CAD build for the part. Positions are in the model's coordinates, mm. A direction names the side the tool comes from. Coordinates: 2 decimals unless noted, no trailing zeros. Order: outer loops, then holes, each group sorted by start corner. A loop starts at its lowest first (then second) coordinate and runs counter-clockwise, first axis right, second up. Notation, with made-up numbers: M 23,9 L 61,9 A20 cw 61,27 Z; hole C -20,71.5 d5. An arc over 180 degrees is marked long. One line per item, written item: value.
from build123d import *

# Parameters (mm, degrees)
F3_D      = 3.3
F3_DEPTH  = 7
F3_TIP    = 0.9914200214
F4_R      = 10
F4_R_2    = 5
F5_DEPTH  = 9.5
F6_SIZE   = 2.5
F8_DEPTH  = 17
F10_D     = 3.3
F10_DEPTH = 5.2
F10_TIP   = 0.9914200214
F11_R     = 4
F12_DEPTH = 0.5
F14_D     = 3.3
F14_DEPTH = 5.2
F14_TIP   = 0.9914200214
F15_R     = 4
F16_DEPTH = 0.5


with BuildPart() as f1:
    # F0 (on Front) → F1 (revolve)
    with BuildSketch(Plane.XZ):
        Polygon((-20, 4), (0, 4), (0, 13), (-18, 13), (-18, 6), (-20, 6), align=None)
    revolve(axis=Axis((-7.6375159387, 0, 0), (-1, 0, 0)))

    # F3
    with Locations(Plane(origin=(-18, 0, 0), x_dir=(0, -1, 0), z_dir=(-1, 0, 0))):
        with Locations((-7, 7), (7, 7), (-7, -7), (7, -7)):
            Hole(F3_D / 2, depth=F3_DEPTH)
            with Locations((0, 0, -(F3_DEPTH + F3_TIP / 2))):  # 118° drill point
                Cone(0, F3_D / 2, F3_TIP, mode=Mode.SUBTRACT)

    # F4 (on face) → F5 (join)
    with BuildSketch(Plane.YZ):
        Circle(F4_R)
        Circle(F4_R_2, mode=Mode.SUBTRACT)
    extrude(amount=F5_DEPTH)

    # F6
    f6_edges = [f1.edges().sort_by_distance(p)[0] for p in [
        (9.5, -10, 0),
    ]]
    chamfer(f6_edges, length=F6_SIZE)

    # F7 (on face) → F8 (cut)
    with BuildSketch(Plane(origin=(-18, 0, 0), x_dir=(0, -1, 0), z_dir=(-1, 0, 0))):
        with BuildLine():
            Line((-4, 12.3693168769), (4, 12.3693168769))
            ThreePointArc((4, 12.3693168769), (0, 13), (-4, 12.3693168769))
        make_face()
        with BuildLine():
            Line((4, -12.3693168769), (-4, -12.3693168769))
            ThreePointArc((-4, -12.3693168769), (0, -13), (4, -12.3693168769))
        make_face()
    extrude(amount=-F8_DEPTH, mode=Mode.SUBTRACT)

    # F10
    with Locations(Plane.XY.offset(12.3693168769)):
        with Locations((-7, 0)):
            Hole(F10_D / 2, depth=F10_DEPTH)
            with Locations((0, 0, -(F10_DEPTH + F10_TIP / 2))):  # 118° drill point
                Cone(0, F10_D / 2, F10_TIP, mode=Mode.SUBTRACT)

    # F11 (on face) → F12 (cut)
    with BuildSketch(Plane.XY.offset(12.3693168769)):
        with Locations((-7, 0)):
            Circle(F11_R)
    extrude(amount=-F12_DEPTH, mode=Mode.SUBTRACT)

    # F14
    with Locations(Plane(origin=(0, 0, -12.3693168769), x_dir=(1, 0, 0), z_dir=(0, 0, -1))):
        with Locations((-7, -0.0519943278)):
            Hole(F14_D / 2, depth=F14_DEPTH)
            with Locations((0, 0, -(F14_DEPTH + F14_TIP / 2))):  # 118° drill point
                Cone(0, F14_D / 2, F14_TIP, mode=Mode.SUBTRACT)

    # F15 (on face) → F16 (cut)
    with BuildSketch(Plane(origin=(0, 0, -12.3693168769), x_dir=(1, 0, 0), z_dir=(0, 0, -1))):
        with Locations((-7, -0.0519943278)):
            Circle(F15_R)
    extrude(amount=-F16_DEPTH, mode=Mode.SUBTRACT)


solid = f1.part
Q1. Drill centre lines: line 1 along Z through (x, y) = (-14.75, -7); line 2 along X through (y, z) = (0, 9.5). Where is each one in solid material? Low to high.
Recorded:
line 1: z = -10.95 to -8.65, -5.35 to 5.35, 8.65 to 10.95
line 2: x = -18 to -8.65, -5.35 to 7.5
Q2. Pin check, flat tips, straight feed: pin 1 Ø5 at (x, z) = (-5, -6) entering from -Y; pin 2 Ø9 at (x, y) = (-7.5, 0.5) entering from -Z; pin 3 Ø4 at (x, y) = (-8, 1.5) entering from +Z; pin 4 Ø5 at (y, z) = (1, -0.5) entering from +X. Stop position of each tip, or through.
Recorded:
pin 1: stops at y = -12.52
pin 2: stops at z = -12.37
pin 3: stops at z = 11.87
pin 4: passes through
Q3. Slice it at C-C (x = -4). List the corners of the cut face in (y, z).
Recorded:
outline: M -4,-12.37 L -2.59,-12.37 L -2.59,-11.87 L 2.7,-11.87 L 2.7,-12.37 L 4,-12.37 A13 ccw 4,12.37 L 2.65,12.37 L 2.65,11.87 L -2.65,11.87 L -2.65,12.37 L -4,12.37 A13 ccw Z; hole C 0,0 d8
Q4. Mould opens along Z. For faces 1 (the face through (-10.2, 6.7, 7.1)), 2 (the face through (-18, -3, -6)), 3 (the face through (-9.126, -11.533, 5.999)) say: released by +Z, released by -Z, zero draft, split by the parting line, or undercut.
Recorded:
face 1: undercut
face 2: zero draft
face 3: split by the parting line
Q5. Which spindle directions (+Z, -Z, +X, -X, +Y, -Y) get a long thin tool onto all of the face, cutting with end or side? Do faces 4 (the face through (-5.35, 0.07, 9.49)), 5 (the face through (-14.45, -8.65, -6.93)), 6 (the face through (0, -8, -7)), 7 (the face through (-14, 0, 12.369)). Say none if no direction does.
Recorded:
face 4: +Z
face 5: -X
face 6: +X
face 7: +Z, -X, +Y, -Y
Q6. Slice it at B-B (z = 0). List the corners of the cut face in (x, y), plus the area to 3 significant figures.
Recorded:
outline: M -20,-6 L -18,-6 L -18,-13 L 0,-13 L 0,-10 L 7,-10 L 9.5,-7.5 L 9.5,-5 L 0,-5 L 0,-4 L -20,-4 Z; M -20,4 L 0,4 L 0,5 L 9.5,5 L 9.5,7.5 L 7,10 L 0,10 L 0,13 L -18,13 L -18,6 L -20,6 Z
area: 421 mm^2
Q7. Slice it at A-A (x = -12.75). List the corners of the cut face in (y, z), plus the area to 3 significant figures.
Recorded:
outline: M -4,-12.37 L 4,-12.37 A13 ccw 4,12.37 L -4,12.37 A13 ccw Z; hole C -7,-7 d3.3; hole C -7,7 d3.3; hole C 0,0 d8; hole C 7,-7 d3.3; hole C 7,7 d3.3
area: 440 mm^2
